Design review of the part built by this model. Coordinates are the model's own, in mm. A direction names the side the tool comes from. Give positions to 0.01 mm unless a question says otherwise; leave off trailing zeros. Order: outer loops, then holes, each group sorted by start corner. A loop starts at its lowest first (then second) coordinate and runs counter-clockwise, first axis right, second up.
```python
from build123d import *

# Parameters (mm, degrees)
SKETCH1_R               = 62
BOSS_EXTRUDE1_DEPTH     = 5
SKETCH2_R               = 2
CUT_EXTRUDE1_DEPTH      = 5
CIRPATTERN1_COUNT       = 2
CIRPATTERN1_ANGLE       = 120
MIRROR1_COPY_1_SKETCH_R = 2
MIRROR1_COPY_1_DEPTH    = 5
SKETCH5_R               = 62
SKETCH5_R_2             = 57
BOSS_EXTRUDE2_DEPTH     = 8
CUT_EXTRUDE2_START      = -90
SKETCH6_R               = 1.25
CUT_EXTRUDE2_DEPTH      = 192
CIRPATTERN2_COUNT       = 2
CIRPATTERN2_ANGLE       = 90


with BuildPart() as part:
    # Sketch1 → Boss-Extrude1 (new body)
    with BuildSketch(Plane(origin=(0, 0, 0), x_dir=(1, 0, 0), z_dir=(0, 1, 0))):
        with Locations(Location((0, 0, 0), (0, 0, 270))):
            Circle(SKETCH1_R)
    extrude(amount=BOSS_EXTRUDE1_DEPTH)

    # Sketch2 → Cut-Extrude1 (cut)
    with BuildSketch(Plane(origin=(0, 5, 0), x_dir=(1, 0, 0), z_dir=(0, 1, 0))):
        with Locations(Location((0, 49.5, 0), (0, 0, 270))):
            Circle(SKETCH2_R)
    cut_extrude1 = extrude(amount=-CUT_EXTRUDE1_DEPTH, mode=Mode.SUBTRACT)

    # CirPattern1: Cut-Extrude1 ×2 about axis
    cirpattern1_axis = Axis((0, 5, 0), (0, 1, 0))
    for i in range(1, CIRPATTERN1_COUNT):
        add(cut_extrude1.rotate(cirpattern1_axis, i * CIRPATTERN1_ANGLE / (CIRPATTERN1_COUNT - 1)), mode=Mode.SUBTRACT)

    # Mirror1: Cut-Extrude1 across plane
    add(cut_extrude1.mirror(Plane(origin=(0, 0, 0), x_dir=(-0.49999999999999806, 0, 0.8660254037844398), z_dir=(-0.8660254037844398, 0, -0.49999999999999806))), mode=Mode.SUBTRACT)

    # Mirror1 copy 1 sketch → Mirror1 copy 1 (cut)
    with BuildSketch(Plane(origin=(0, 5, 0), x_dir=(1, 0, 0), z_dir=(0, 1, 0))):
        with Locations((0, -49.5)):
            Circle(MIRROR1_COPY_1_SKETCH_R)
    extrude(amount=-MIRROR1_COPY_1_DEPTH, mode=Mode.SUBTRACT)

    # Sketch5 → Boss-Extrude2 (add)
    with BuildSketch(Plane(origin=(0, 5, 0), x_dir=(1, 0, 0), z_dir=(0, 1, 0))):
        with Locations(Location((0, 0, 0), (0, 0, 270))):
            Circle(SKETCH5_R)
        with Locations(Location((0, 0, 0), (0, 0, 270))):
            Circle(SKETCH5_R_2, mode=Mode.SUBTRACT)
    extrude(amount=BOSS_EXTRUDE2_DEPTH)

    # Sketch6 → Cut-Extrude2 (cut)
    with BuildSketch(Plane(origin=(0, 0, 0), x_dir=(-0.49999999999999806, 0, 0.8660254037844398), z_dir=(-0.8660254037844398, 0, -0.49999999999999806)).offset(CUT_EXTRUDE2_START)):
        with Locations(Location((0, 7, 0), (0, 0, 180))):
            Circle(SKETCH6_R)
    cut_extrude2 = extrude(amount=CUT_EXTRUDE2_DEPTH, mode=Mode.SUBTRACT)

    # CirPattern2: Cut-Extrude2 ×2 about axis
    cirpattern2_axis = Axis((0, 13, 0), (0, 1, 0))
    for i in range(1, CIRPATTERN2_COUNT):
        add(cut_extrude2.rotate(cirpattern2_axis, i * CIRPATTERN2_ANGLE / (CIRPATTERN2_COUNT - 1)), mode=Mode.SUBTRACT)


solid = part.part
```
1. For line 1 along X through (y, z) = (9, 0); line 2 along Z through (x, y) = (52, 6.75); line 3 along Y through (x, z) = (-16, 26), list the stretches that pass through material, from the lowest coordinate up.
Recorded:
line 1: x = -62 to -57, 57 to 62
line 2: z = -33.76 to -23.35, 23.35 to 28.61, 31.44 to 33.76
line 3: y = 0 to 5
2. Take a section at D-D (z = 17). State the section outline as (x, y) points, then the cut area to 3 significant figures.
Recorded:
outline: (-59.62, 0) - (59.62, 0) - (59.62, 13) - (54.41, 13) - (54.41, 5) - (-54.41, 5) - (-54.41, 13) - (-59.62, 13) - close
area: 680 mm2
3. Take a section at C-C (y = 3.5). State the section outline as (x, z) points.
Recorded:
outline: circle Ø124 at (0, 0); hole circle Ø4 at (-42.87, 24.75); hole circle Ø4 at (0, -49.5); hole circle Ø4 at (0, 49.5); hole circle Ø4 at (42.87, -24.75)
4. Take a section at B-B (z = 0). State the section outline as (x, y) points.
Recorded:
outline: (-62, 0) - (62, 0) - (62, 13) - (57, 13) - (57, 5) - (-57, 5) - (-57, 13) - (-62, 13) - close
5. Take a section at A-A (x = 0). State the section outline as (y, z) points, then the cut area to 3 significant figures.
Recorded:
outline: (0, -62) - (13, -62) - (13, -57) - (5, -57) - (5, -51.5) - (0, -51.5) - close; (0, -47.5) - (5, -47.5) - (5, 47.5) - (0, 47.5) - close; (0, 51.5) - (5, 51.5) - (5, 57) - (13, 57) - (13, 62) - (0, 62) - close
area: 660 mm2
6. Machinability: for faces 4 (the face through (-52.12, 6.95, -28.65)), 5 (the face through (-55.645, 8.944, -12.356)), which of the approach directions +Z, -Z, +X, -X, +Y, -Y give a long, thin tool a straight path to every point of the face, cutting with its end or side? Answer none if there is none.
Recorded:
face 4: none
face 5: +Y
7. For pin 1 (8 mm diameter, centred on x = -13, z = 41.5, fed in from +Y); pin 2 (3 mm diameter, centred on x = 0, z = 49.5, fed in from +Y); pin 3 (2 mm diameter, centred on x = 13.5, y = 4, fed in from +Z); pin 4 (6 mm diameter, centred on y = 4.5, z = 4.5, fed in from -X), all flat-tipped, find the tip position at first contact; note any pin that passes through.
Recorded:
pin 1: stops at y = 5
pin 2: passes through
pin 3: stops at z = 60.73
pin 4: stops at x = -61.98
8. Draft analysis for pull direction Z (two halves, no side actions). For faces 1 (the face through (61.472, 6.409, -8.071)), 2 (the face through (-27.27, 13, 50.23)), 3 (the face through (0.923, 2.535, 51.274)), state which applies: pulls with the +Z half, pulls with the -Z half, needs draft (parallel to the pull), parting line crosses it, or undercut.
Recorded:
face 1: parting line crosses it
face 2: needs draft
face 3: undercut
